from build123d import *

# Parameters (mm, degrees)
TROU_TARAUD_M14X1_51_D     = 14
TROU_TARAUD_M14X1_51_DEPTH = 12
TROU_TARAUD_M14X1_51_TIP   = 4.206024333
TROU_TARAUD_M61_AT_2_COUNT = 2
TROU_TARAUD_M61_AT_2_PITCH = 20


with BuildPart() as part:
    # Esquisse1 → Révolution1 (revolve)
    with BuildSketch(Plane.XY, mode=Mode.PRIVATE) as r_volution1_sk:
        Polygon((-6.5, 31), (-3, 31), (-3, 0), (-10, 0), (-10, 15), (-6.5, 15), align=None)
    revolve(r_volution1_sk.sketch.rotate(Axis((0, 39.529907563, 0), (0, -1, 0)), 270), axis=Axis((0, 39.529907563, 0), (0, -1, 0)))

    # Trou taraudé M14x1.51
    with Locations(Plane(origin=(0, 0, 0), x_dir=(-1, 0, 0), z_dir=(0, -1, 0))):
        with Locations((0, 0)):
            Hole(TROU_TARAUD_M14X1_51_D / 2, depth=TROU_TARAUD_M14X1_51_DEPTH)
            with Locations((0, 0, -(TROU_TARAUD_M14X1_51_DEPTH + TROU_TARAUD_M14X1_51_TIP / 2))):  # 118° drill point
                Cone(0, TROU_TARAUD_M14X1_51_D / 2, TROU_TARAUD_M14X1_51_TIP, mode=Mode.SUBTRACT)

    # Esquisse7 → Trou taraudé M61 (revolve, cut)
    with BuildSketch(Plane(origin=(0, 6, 0), x_dir=(0, 1, 0), z_dir=(1, 0, 0))):
        Polygon((0, 0), (0, 17.502151548), (2.5, 16), (2.5, 0), align=None)
    trou_taraud_m61 = revolve(axis=Axis((0, 6, -6.35), (0, 0, 1)), mode=Mode.SUBTRACT)

    # Trou taraudé M61 at 2: Trou taraudé M61 ×2
    with Locations(*[(0, i * TROU_TARAUD_M61_AT_2_PITCH, 0) for i in range(1, TROU_TARAUD_M61_AT_2_COUNT)]):
        add(trou_taraud_m61, mode=Mode.SUBTRACT)


solid = part.part
Work out the finished part from the listing and answer in its coordinate system (mm). A direction names the side the tool comes from. Round coordinates to 2 decimals unless told otherwise and drop trailing zeros. Loops run counter-clockwise (first coordinate to the right, second up) from the corner with the lowest first, then second, coordinate; pieces in that order, holes last. Notation, with made-up numbers: (57.25, 60.5) -> (100.25, 60.5) arc R19 cw to (100.25, 91.5) -> close; hole circle Ø5 at (39.5, 47). An arc over 180 degrees is marked (long way). Use one line per item in the form item = value.
(1) Find section C-C on x = -1.75. Give the number of separate pieces and of enclosed holes in the cut face, then the cut area to 3 significant figures.
Answer list:
separate_pieces = 4
enclosed_holes = 0
area = 205 mm2
(2) A tool of negligible diameter and unlimited length cuts with its end or side. For faces 4 (the cylindrical face through (3.763, 6.084, -5.902)), 5 (the cylindrical face through (-0.751, 8.385, 8.245)), 6 (the cylindrical face through (3.955, 23.112, -5.158)), from which of +Z, -Z, +X, -X, +Y, -Y can it reach the whole face along a straight path? Write none if from no direction.
Answer list:
face_4 = -Y
face_5 = +Z
face_6 = +Y
(3) Find section A-A on z = 0. Give the vertices of the cut face in (x, y), then the cut area to 3 significant figures.
Answer list:
outline = (-10, 0) -> (-7, 0) -> (-7, 12) -> (-3, 14.4) -> (-3, 31) -> (-6.5, 31) -> (-6.5, 15) -> (-10, 15) -> close; (3, 14.4) -> (7, 12) -> (7, 0) -> (10, 0) -> (10, 15) -> (6.5, 15) -> (6.5, 31) -> (3, 31) -> close
area = 216 mm2
(4) For a pull along X with two mould halves and no side action, classify faces 1 (the flat face through (1, 31, 3)), 2 (the cylindrical face through (9.76, 7.6, -2.17)), 3 (the cylindrical face through (0.96, 28.31, 4.05)) as released by +X, released by -X, zero draft, split by the parting line, or undercut.
Answer list:
face_1 = zero draft
face_2 = split by the parting line
face_3 = undercut
(5) Straight lines are drawn through the part: line 1 (X direction, y = 4, z = -1); line 2 (X direction, y = 6, z = 8.7); line 3 (Y direction, x = 8, z = -0.5). For each, find the intervals that lie inside material, in ascending order.
Answer list:
line_1 = -9.95 to -6.93, 6.93 to 9.95
line_2 = -4.93 to -2.5, 2.5 to 4.93
line_3 = 0 to 15
(6) Find section B-B on y = 20. Give the vertices of the cut face in (x, z).
Answer list:
outline = circle Ø13 at (0, 0); hole circle Ø6 at (0, 0)
(7) Find section D-D on y = 26. Give the vertices of the cut face in (x, z).
Answer list:
outline = (-2.5, 1.66) -> (-2.5, 6) arc R6.5 ccw (long way) to (2.5, 6) -> (2.5, 1.66) arc R3 cw (long way) to start
(8) Flat-ended cylindrical pins translate along their axes: P1, Ø1.5, axis at y = 23.5, z = -2.5, coming from the +X side; P2, Ø5, axis at y = 18.5, z = 1.5, coming from the -X side; P3, Ø8, axis at x = -5, y = 24, coming from the -Z side; P4, Ø3, axis at x = -4, z = -4.5, coming from the -Y side. Find the tip coordinate at first contact, or state that the pin passes through.
Answer list:
P1 = 6.26
P2 = -6.5
P3 = -6.42
P4 = 0
